```python
from build123d import *

# Parameters (mm, degrees)
CROQUIS1_W              = 10
CROQUIS1_H              = 3
SALIENTE_EXTRUIR1_DEPTH = 3


with BuildPart() as part:
    # Croquis1 → Saliente-Extruir1 (new body)
    with BuildSketch(Plane(origin=(0, 0, 0), x_dir=(0, 0, -1), z_dir=(1, 0, 0))):
        Polygon((-60.530143817, -78.620199336), (-40.530143817, -78.620199336), (-40.530143817, -81.620199336), (-20.530143817, -81.620199336), (-20.530143817, -78.620199336), (-0.530143817, -78.620199336), (-0.530143817, -81.620199336), (19.469856183, -81.620199336), (19.469856183, -78.620199336), (39.469856183, -78.620199336), (39.469856183, -81.620199336), (59.469856183, -81.620199336), (59.469856183, 11.086867688), (-60.530143817, 11.086867688), align=None)
        with Locations((14.469856183, -57.120199336)):
            Rectangle(CROQUIS1_W, CROQUIS1_H, mode=Mode.SUBTRACT)
    extrude(amount=SALIENTE_EXTRUIR1_DEPTH)


solid = part.part
```
The listing builds one solid part. Answer for the finished solid, in the listing's coordinates (mm). A direction names the side the tool comes from. Give positions to 0.01 mm unless a question says otherwise; leave off trailing zeros. Order: outer loops, then holes, each group sorted by start corner. A loop starts at its lowest first (then second) coordinate and runs counter-clockwise, first axis right, second up. Notation, with made-up numbers: M 56.25,-16.75 L 84.25,-16.75 A31 cw 84.25,17.25 Z; hole C 46,-35.5 d9. An arc over 180 degrees is marked long. Put each result on its own line as item: value. Start each with the question number.
Item 1: Find the intervals of material crossed by line 1 along Y through (x, z) = (2.7, -16); line 2 along Y through (x, z) = (1, 4), in increasing order.
Item 2: The part is cut by section A-A, the plane x = 0.5. Determine the outline of the cut face in (y, z).
Item 3: Which of the six approach directions +Z, -Z, +X, -X, +Y, -Y give full straight-line access (tool end or side, diameter ignored) to faces 1 (the face through (1, -81.62, 31)), 2 (the face through (1, -80, -19.47)), 3 (the face through (1, -78.62, 51)), 4 (the face through (1, -57, -19.47)), 5 (the face through (1, -36, -59.47))?
Item 4: Flat-ended cylindrical pins translate along their axes: P1, Ø1.5, axis at x = 1.5, y = -79.5, coming from the +Z side; P2, Ø1.5, axis at x = 1.5, z = 50.5, coming from the -Y side. Find the tip coordinate at first contact, or state that the pin passes through.
Item 5: For a pull along Y with two mould halves and no side action, classify faces 6 (the face through (1, -57, -9.47)), 7 (the face through (1, -80, 0.53)), 8 (the face through (1, -81.62, -49)), 9 (the face through (1, 11.087, 0)) as +Y half, -Y half, draft (parallel to the pull), parting line (faces both ways), or undercut.
Item 6: The part is cut by section B-B, the plane z = 42. Determine the outline of the cut face in (x, y).
Answer key:
1. line 1: y = -81.62 to -58.62, -55.62 to 11.09
1. line 2: y = -78.62 to 11.09
2. outline: M -81.62,-59.47 L 11.09,-59.47 L 11.09,60.53 L -78.62,60.53 L -78.62,40.53 L -81.62,40.53 L -81.62,20.53 L -78.62,20.53 L -78.62,0.53 L -81.62,0.53 L -81.62,-19.47 L -78.62,-19.47 L -78.62,-39.47 L -81.62,-39.47 Z; hole M -58.62,-19.47 L -55.62,-19.47 L -55.62,-9.47 L -58.62,-9.47 Z
3. face 1: +Z, -Z, +X, -X, -Y
3. face 2: +X, -X, -Y
3. face 3: +Z, +X, -X, -Y
3. face 4: +X, -X
3. face 5: -Z, +X, -X, +Y, -Y
4. P1: stops at z = 40.53
4. P2: stops at y = -78.62
5. face 6: undercut
5. face 7: draft
5. face 8: -Y half
5. face 9: +Y half
6. outline: M 0,-78.62 L 3,-78.62 L 3,11.09 L 0,11.09 Z
